Autodesk Inventor part; units mm, degrees
ref_plane "YZ Plane" through (0, 0, 0) normal (1, 0, 0) x (0, 1, 0)
ref_plane "XZ Plane" through (0, 0, 0) normal (0, 1, 0) x (-1, 0, 0)
ref_plane "XY Plane" through (0, 0, 0) normal (0, 0, 1) x (1, 0, 0)
sketch "Эскиз1" plane through (0, 0, 0) normal (0, 0, 1) x (1, 0, 0)
  line L0 (-2.3094, 4) -> (2.3094, 4)
  line L1 (2.3094, 4) -> (4.6188, 0)
  line L2 (4.6188, 0) -> (2.3094, -4)
  line L3 (2.3094, -4) -> (-2.3094, -4)
  line L4 (-2.3094, -4) -> (-4.6188, 0)
  line L5 (-4.6188, 0) -> (-2.3094, 4)
  point P0 (0, 0)
  point P1 (0, 0)
  dimension "d0" = 8
extrude "Выдавливание1" add sketch "Эскиз1" along normal blind 4
sketch "Эскиз2" plane through (0, 0, 4) normal (0, 0, 1) x (1, 0, 0)
  circle A0 centre (0, 0) radius 2.5
  dimension "d3" = 5
extrude "Выдавливание2" add sketch "Эскиз2" along normal blind 30
fillet "Сопряжение1" radius 0.6 6 edges at (-2.3094, -4, 2) (2.3094, -4, 2) (4.6188, 0, 2) (2.3094, 4, 2) (-2.3094, 4, 2) (-4.6188, 0, 2)
chamfer "Фаска1" distance 0.4 angle 45 26 edges at (3.4641, 2, 4) (2.263, 3.9196, 4) (0, 4, 4) (-2.263, 3.9196, 4) (-3.4641, 2, 4) (-4.526, 0, 4) (-3.4641, -2, 4) (-2.263, -3.9196, 4) (0, -4, 4) (2.263, -3.9196, 4) (3.4641, -2, 4) (4.526, 0, 4) (-3.4641, 2, 0) (-4.526, 0, 0) (-3.4641, -2, 0) (-2.263, -3.9196, 0) (0, -4, 0) (2.263, -3.9196, 0) (3.4641, -2, 0) (4.526, 0, 0) (3.4641, 2, 0) (2.263, 3.9196, 0) (0, 4, 0) (-2.263, 3.9196, 0) (-2.5, 0, 34) (-2.5, 0, 4)
thread "Резьба1"
properties part number "Болт М5х30"
Work out the finished part from the listing and answer in its coordinate system (mm). A direction names the side the tool comes from. Give positions to 0.01 mm unless a question says otherwise; leave off trailing zeros. Write each loop counter-clockwise with the first axis right and the second up, starting at its lowest first coordinate (ties: lowest second). Pieces come first, ordered by that corner, then holes. Notation, with made-up numbers: (-22.5, 56.5) -> (28.5, 56.5) arc R21 cw to (28.5, 63.5) -> close; hole circle Ø9 at (7, 12.25). An arc over 180 degrees is marked (long way). Write item = value, one per line.
Q1. Section C-C on x = -3.25 is taken. Determine the outline of the cut face in (y, z).
Computed values:
outline = (-2.37, 0.4) -> (-1.57, 0) -> (1.57, 0) -> (2.37, 0.4) -> (2.37, 3.6) -> (1.57, 4) -> (-1.57, 4) -> (-2.37, 3.6) -> close
Q2. Section B-B on z = 17.5 is taken. Determine the outline of the cut face in (x, y).
Computed values:
outline = circle Ø5 at (0, 0)
Q3. Consider line 1 along Z through (x, y) = (2.25, -2); line 2 along Y through (x, z) = (-0.75, 15.5); line 3 along Y through (x, z) = (-3, 3.5). Determine where each line is inside the solid, lowest interval first.
Computed values:
line_1 = 0 to 4
line_2 = -2.38 to 2.38
line_3 = -2.8 to 2.8
Q4. Flat-ended cylindrical pins translate along their axes: pin 1 Ø1.5 at (x, y) = (-2, 2) entering from -Z; pin 2 Ø2 at (y, z) = (2.5, 7.5) entering from +X. Find the tip coordinate at first contact, or state that the pin passes through.
Computed values:
pin_1 = 0
pin_2 = 2
Q5. Section A-A on x = 0 is taken. Determine the outline of the cut face in (y, z).
Computed values:
outline = (-4, 0.4) -> (-3.6, 0) -> (3.6, 0) -> (4, 0.4) -> (4, 3.6) -> (3.6, 4) -> (2.9, 4) -> (2.5, 4.4) -> (2.5, 33.6) -> (2.1, 34) -> (-2.1, 34) -> (-2.5, 33.6) -> (-2.5, 4.4) -> (-2.9, 4) -> (-3.6, 4) -> (-4, 3.6) -> close
Q6. A tool of negligible diameter and unlimited length cuts with its end or side. For faces 1 (the cylindrical face through (-0.54, 2.44, 18.8)), 2 (the flat face through (-3.28, -1.925, 3.797)), from which of +Z, -Z, +X, -X, +Y, -Y can it reach the whole face along a straight path? Write none if from no direction.
Computed values:
face_1 = +Z
face_2 = +Z, -X, -Y
